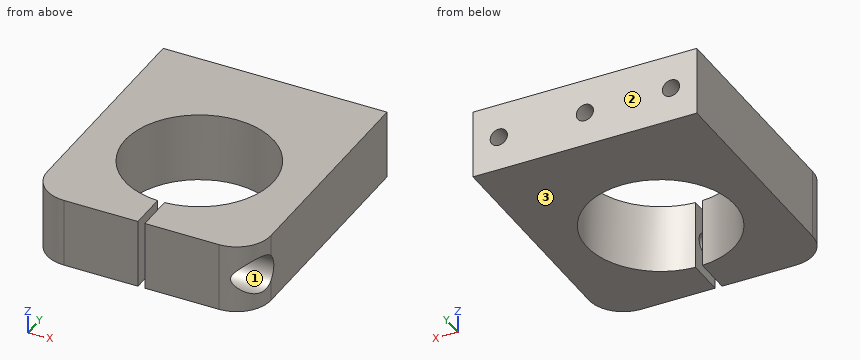
from build123d import *

# Parameters (mm, degrees)
AUFSATZ_LINEAR_AUSTRAGEN1_DEPTH = 20
M6_GEWINDEBOHRUNG1_D            = 5
M6_GEWINDEBOHRUNG1_DEPTH        = 17
M6_GEWINDEBOHRUNG1_TIP          = 1.502151548
SKIZZE4_R                       = 3
SCHNITT_LINEAR_AUSTRAGEN1_DEPTH = 40
SCHNITT_LINEAR_START            = 20
SKIZZE5_R                       = 5.5
SCHNITT_LINEAR_AUSTRAGEN2_DEPTH = 20


with BuildPart() as part:
    # Skizze1 → Aufsatz-Linear austragen1 (new body)
    with BuildSketch(Plane.XY):
        with BuildLine():
            Line((-32.5, 42.5), (32.5, 42.5))
            Line((32.5, 42.5), (32.5, -22.5))
            ThreePointArc((32.5, -22.5), (29.571067812, -29.571067812), (22.5, -32.5))
            Line((22.5, -32.5), (1, -32.5))
            Line((1, -32.5), (1, -21.476731595))
            ThreePointArc((1, -21.476731595), (0, 21.5), (-1, -21.476731595))
            Line((-1, -21.476731595), (-1, -32.5))
            Line((-1, -32.5), (-22.5, -32.5))
            ThreePointArc((-22.5, -32.5), (-29.571067812, -29.571067812), (-32.5, -22.5))
            Line((-32.5, -22.5), (-32.5, 42.5))
        make_face()
    extrude(amount=AUFSATZ_LINEAR_AUSTRAGEN1_DEPTH)

    # M6 Gewindebohrung1
    with Locations(Plane(origin=(0, 42.5, 0), x_dir=(1, 0, 0), z_dir=(0, 1, 0))):
        with Locations((-25, -10), (0, -10), (25, -10)):
            Hole(M6_GEWINDEBOHRUNG1_D / 2, depth=M6_GEWINDEBOHRUNG1_DEPTH)
            with Locations((0, 0, -(M6_GEWINDEBOHRUNG1_DEPTH + M6_GEWINDEBOHRUNG1_TIP / 2))):  # 118° drill point
                Cone(0, M6_GEWINDEBOHRUNG1_D / 2, M6_GEWINDEBOHRUNG1_TIP, mode=Mode.SUBTRACT)

    # Skizze4 → Schnitt-Linear austragen1 (cut)
    with BuildSketch(Plane(origin=(0, 0, 0), x_dir=(0, 0, -1), z_dir=(1, 0, 0))):
        with Locations(Location((-10, -26.5, 0), (0, 0, 180))):
            Circle(SKIZZE4_R)
    extrude(amount=SCHNITT_LINEAR_AUSTRAGEN1_DEPTH, mode=Mode.SUBTRACT)

    # Skizze5 → Schnitt-Linear austragen2 (cut)
    with BuildSketch(Plane(origin=(0, 0, 0), x_dir=(0, 0, -1), z_dir=(1, 0, 0)).offset(SCHNITT_LINEAR_START)):
        with Locations(Location((-10, -26.5, 0), (0, 0, 133.341758227))):
            Circle(SKIZZE5_R)
    extrude(amount=SCHNITT_LINEAR_AUSTRAGEN2_DEPTH, mode=Mode.SUBTRACT)


solid = part.part
Could you check a few things on this model? Use its own coordinates, in mm. Face numbers are marked on the shaded views. Give positions to 0.01 mm unless a question says otherwise; leave off trailing zeros. Write each loop counter-clockwise with the first axis right and the second up, starting at its lowest first coordinate (ties: lowest second). Pieces come first, ordered by that corner, then holes. Notation, with made-up numbers: (16.5, -35.5) -> (32.5, -35.5) arc R5 cw to (32.5, -30.5) -> close; hole circle Ø10 at (52, 76.25). An arc over 180 degrees is marked (long way). Write each question's results on one line, items separated by ' | '. Start each with the question number.
Q1. I need wall thicknesses on probe 1 along X at (y, z) = (31.25, 10); probe 2 along Y at (x, z) = (8, 10); probe 3 along Z at (x, y) = (0, 33). Which ranges of each line are inside material? Lowest first, please.
Q2. Suppose I cut it at D-D, the plane x = -18.5. List the corners of the cut face in (y, z) for me.
Q3. Suppose I cut it at B-B, the plane z = 2.75. List the corners of the cut face in (x, y) for me, and give its area (3 significant figures).
Q4. I'm going to push flat-ended pins straight in: pin 1 Ø6 at (x, z) = (-24.5, 17) entering from -Y; pin 2 Ø3.5 at (y, z) = (-24, 7.5) entering from +X; pin 3 Ø3 at (x, z) = (-25, 10) entering from +Y; pin 4 Ø9 at (y, z) = (-28, 6.5) entering from -X. Where does each tip first touch, or does it pass through?
Q5. Suppose I cut it at A-A, the plane y = 0. List the corners of the cut face in (x, z) for me.
Q6. Suppose I cut it at C-C, the plane y = 33.5. List the corners of the cut face in (x, z) for me.
Q7. We'd pull the mould along Z, two halves only. Please class the marked faces 1, 2 and 3: +Z half, -Z half, draft (parallel to the pull), parting line (faces both ways), or undercut.
Outcome:
1) probe 1: -32.5 to -27.5, -22.5 to -2.5, 2.5 to 22.5, 27.5 to 32.5 | probe 2: -32.5 to -29.5, -23.5 to -19.96, 19.96 to 42.5 | probe 3: 0 to 7.5, 12.5 to 20
2) outline: (-32.5, 0) -> (-10.95, 0) -> (-10.95, 20) -> (-32.5, 20) -> close; (10.95, 0) -> (42.5, 0) -> (42.5, 20) -> (10.95, 20) -> close
3) outline: (-32.5, -22.5) arc R10 ccw to (-22.5, -32.5) -> (-1, -32.5) -> (-1, -21.48) arc R21.5 cw (long way) to (1, -21.48) -> (1, -32.5) -> (22.5, -32.5) arc R10 ccw to (32.5, -22.5) -> (32.5, 42.5) -> (-32.5, 42.5) -> close | area: 3,360 mm2
4) pin 1: y = -32.5 | pin 2: x = 20 | pin 3: y = 24.9 | pin 4: x = -32.45
5) outline: (-32.5, 0) -> (-21.5, 0) -> (-21.5, 20) -> (-32.5, 20) -> close; (21.5, 0) -> (32.5, 0) -> (32.5, 20) -> (21.5, 20) -> close
6) outline: (-32.5, 0) -> (32.5, 0) -> (32.5, 20) -> (-32.5, 20) -> close; hole circle Ø5 at (-25, 10); hole circle Ø5 at (0, 10); hole circle Ø5 at (25, 10)
7) face 1: undercut | face 2: draft | face 3: -Z half
